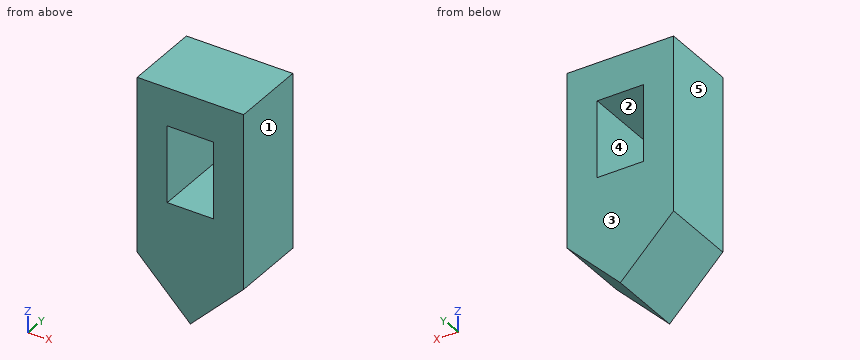
from build123d import *

# Parameters (mm, degrees)
SKETCH2_W           = 7
SKETCH2_H           = 15
SKETCH2_W_2         = 3.05
SKETCH2_H_2         = 5.05
BOSS_EXTRUDE1_DEPTH = 5
CHAMFER1_SIZE       = 3.5


with BuildPart() as part:
    # Sketch2 → Boss-Extrude1 (new body)
    with BuildSketch(Plane(origin=(0, 0, 0), x_dir=(1, 0, 0), z_dir=(0, 1, 0))):
        with Locations((3.5, 7.5)):
            Rectangle(SKETCH2_W, SKETCH2_H)
        with Locations((3.5, 5.025)):
            Rectangle(SKETCH2_W_2, SKETCH2_H_2, mode=Mode.SUBTRACT)
    extrude(amount=BOSS_EXTRUDE1_DEPTH)

    # Chamfer1
    chamfer1_edges = [part.edges().sort_by_distance(p)[0] for p in [
        (0, 2.5, -15),
        (7, 2.5, -15),
    ]]
    chamfer(chamfer1_edges, length=CHAMFER1_SIZE - 0.0001)  # a hair under: the kernel refuses the full size


solid = part.part
Can you work these out from the model? Positions are in its coordinate system, mm. Face numbers are marked on the shaded views. A direction names the side the tool comes from. Coordinates: 2 decimals unless noted, no trailing zeros. Order: outer loops, then holes, each group sorted by start corner. A loop starts at its lowest first (then second) coordinate and runs counter-clockwise, first axis right, second up. Notation, with made-up numbers: (69.5, 41) - (91.5, 41) arc R17 cw to (91.5, 47) - close; hole circle Ø8 at (-2.75, -3). An arc over 180 degrees is marked (long way). Answer as a JSON object with one key per item and string values. Group by question number.
Q1. On a 3-axis mill with a long thin cutter (end or side, diameter ignored), from which of +Z, -Z, +X, -X, +Y, -Y can I reach the whole of each face in a straight line? I mean the marked faces 4 and 5. Say none if no direction works.
Q2. Imagine slicing it at C-C (x = 4.25). Please give me the cut outline in (y, z), and give its area (3 significant figures).
Q3. Imagine slicing it at A-A (z = -4.5). Please give me the cut outline in (x, y) (3 decimals).
Q4. I need wall thicknesses on line 1 (X direction, y = 1.35, z = -5.75) (3 decimals); line 2 (Z direction, x = 2.25, y = 2.4); line 3 (Z direction, x = 3.25, y = 0.45). Which ranges of each line are inside material? Lowest first, please. Write a range as from..to.
Q5. Imagine slicing it at D-D (x = 5.25). Please give me the cut outline in (y, z).
Q6. Will this pin go through, and if not, where does the flat tip stop? P1, Ø1.5, axis at x = 3, y = 1.5, coming from the -Z side.
Q7. We'd pull the mould along X, two halves only. Please class the marked faces 1, 2 and 3: +X half, -X half, draft (parallel to the pull), parting line (faces both ways), or undercut.
Determined:
{
 "1": {"face 4": "+Y, -Y", "face 5": "+Z, -Z, -X, +Y, -Y"},
 "2": {"outline": "(0, -14.25) - (5, -14.25) - (5, -7.55) - (0, -7.55) - close; (0, -2.5) - (5, -2.5) - (5, 0) - (0, 0) - close", "area": "46.0 mm2"},
 "3": {"outline": "(0, 0) - (1.975, 0) - (1.975, 5) - (0, 5) - close; (5.025, 0) - (7, 0) - (7, 5) - (5.025, 5) - close"},
 "4": {"line 1": "x = 0..1.975, 5.025..7", "line 2": "z = -13.75..-7.55, -2.5..0", "line 3": "z = -14.75..-7.55, -2.5..0"},
 "5": {"outline": "(0, -13.25) - (5, -13.25) - (5, 0) - (0, 0) - close"},
 "6": {"P1": "stops at z = -15"},
 "7": {"face 1": "+X half", "face 2": "undercut", "face 3": "draft"}
}
